Could you check a few things on this model? Use its own coordinates, in mm. Coordinates: 2 decimals unless noted, no trailing zeros. Loops run counter-clockwise (first coordinate to the right, second up) from the corner with the lowest first, then second, coordinate; pieces in that order, holes last. Notation, with made-up numbers: (0, -25) - (13, -25) arc R16 ccw to (13, -11) - close; hole circle Ø9 at (-21, -37.5). An arc over 180 degrees is marked (long way). Use CSV: the item, a comma, the result in double quotes.
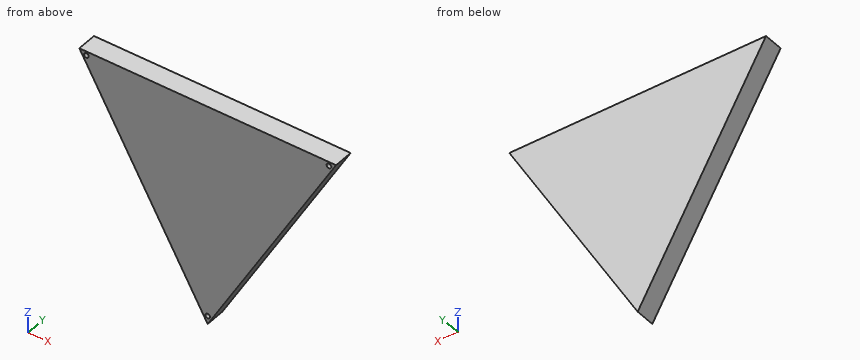
from build123d import *

# Parameters (mm, degrees)
BOSS_EXTRUDE1_DEPTH = 17
SKETCH3_R           = 2
CUT_EXTRUDE2_DEPTH  = 14


with BuildPart() as part:
    # Sketch2 → Boss-Extrude1 (new body)
    with BuildSketch(Plane(origin=(0, 0, 0), x_dir=(1, 0, 0), z_dir=(0, 1, 0))):
        Polygon((-41.583286951, 150.67482391), (-151.583286951, -39.850764923), (68.416713049, -39.850764923), align=None)
    extrude(amount=BOSS_EXTRUDE1_DEPTH)

    # Sketch3 → Cut-Extrude2 (cut)
    with BuildSketch(Plane.XZ):
        with Locations(Location((-145.521109124, 36.350764923, 0), (0, 0, 270))):
            Circle(SKETCH3_R)
        with Locations(Location((62.354535223, 36.350764923, 0), (0, 0, 270))):
            Circle(SKETCH3_R)
        with Locations(Location((-41.583286951, -143.67482391, 0), (0, 0, 270))):
            Circle(SKETCH3_R)
    extrude(amount=-CUT_EXTRUDE2_DEPTH, mode=Mode.SUBTRACT)


solid = part.part
(1) Will these pins go through, and if not, where does the flat tip stop? pin 1 (12 mm diameter, centred on x = -125, z = -17.5, fed in from -Y); pin 2 (1.5 mm diameter, centred on y = 5.5, z = -23, fed in from -X); pin 3 (2 mm diameter, centred on x = 41, y = 13, fed in from -Z); pin 4 (1.2 mm diameter, centred on x = -146.5, z = 36, fed in from -Y).
Computed:
pin 1,"stops at y = 0"
pin 2,"stops at x = -115.73"
pin 3,"stops at z = -9.37"
pin 4,"stops at y = 14"
(2) Suppose I cut it at C-C (x = -56). Write out the boundary of the cut face in (y, z).
Computed:
outline,"(0, -125.7) - (17, -125.7) - (17, 39.85) - (0, 39.85) - close"
(3) Suppose I cut it at A-A (y = 11). Write out the boundary of the cut face in (x, z), plus the area to 3 significant figures.
Computed:
outline,"(-151.58, 39.85) - (-41.58, -150.67) - (68.42, 39.85) - close; hole circle Ø4 at (-145.52, 36.35); hole circle Ø4 at (-41.58, -143.67); hole circle Ø4 at (62.35, 36.35)"
area,"20,900 mm²"
(4) Suppose I cut it at B-B (z = -38). Write out the boundary of the cut face in (x, y).
Computed:
outline,"(-106.64, 0) - (23.47, 0) - (23.47, 17) - (-106.64, 17) - close"
(5) Please list where these lines run through material, in increasing order: line 1 (X direction, y = 11.25, z = -53); line 2 (X direction, y = 8.5, z = 30); line 3 (Z direction, x = -133.5, y = 10.5).
Computed:
line 1,"x = -97.98 to 14.81"
line 2,"x = -145.9 to 62.73"
line 3,"z = 8.53 to 39.85"
